Here's how the part is built. I have some questions about the finished solid (model axes, mm). A direction names the side the tool comes from. Round coordinates to 2 decimals unless told otherwise and drop trailing zeros. Loops run counter-clockwise (first coordinate to the right, second up) from the corner with the lowest first, then second, coordinate; pieces in that order, holes last. Notation, with made-up numbers: M -18.75,10 L 28.25,10 A20 ccw 28.25,49 Z; hole C 19,1 d7. An arc over 180 degrees is marked long. Answer as a JSON object with one key per item and string values.
Autodesk Inventor part; units mm, degrees
ref_plane "YZ Plane" through (0, 0, 0) normal (1, 0, 0) x (0, 1, 0)
ref_plane "XZ Plane" through (0, 0, 0) normal (0, 1, 0) x (-1, 0, 0)
ref_plane "XY Plane" through (0, 0, 0) normal (0, 0, 1) x (1, 0, 0)
sketch "Sketch1" plane through (0, 0, 0) normal (0, 0, 1) x (1, 0, 0)
  line L0 (0, 0) -> (55, 0)
  line L1 (55, 0) -> (55, 10)
  line L2 (55, 10) -> (0, 10)
  line L3 (0, 10) -> (0, 0)
  dimension "d0" = 55
  dimension "d1" = 10
extrude "Extrusion1" add sketch "Sketch1" along normal blind 3.175
sketch "Sketch3" plane through (0, 0, 3.175) normal (0, 0, 1) x (1, 0, 0)
  line L0 (37, 5) -> (55, 5)
  line L1 (0, 10) -> (55, 10)
  line L2 (0, 0) -> (6, 0) construction
  line L3 (6, 0) -> (6, 10) construction
  line L4 (6, 10) -> (0, 10) construction
  line L5 (0, 10) -> (0, 0) construction
  line L6 (-4.3576, 5) -> (33.1549, 5) construction
  line L7 (6, 0) -> (28.9, 0) construction
  line L8 (28.9, 0) -> (28.9, 6.8677) construction
  line L9 (28.9, 6.8677) -> (6, 6.8677) construction
  line L10 (6, 6.8677) -> (6, 0) construction
  point P0 (6, 5)
  point P1 (28.9, 5)
  dimension "d8" = 6
  dimension "d9" = 22.9
hole "Hole1" at (6, 5, 3.175) at (28.9, 5, 3.175) direction (0, 0, -1) diameter 3.2 end through all
sketch "Sketch6" plane through (0, 0, 3.175) normal (0, 0, 1) x (1, 0, 0)
  line L0 (55, 10) -> (37, 10)
  line L1 (37, 10) -> (37, 5)
  line L2 (37, 5) -> (55, 5)
  line L3 (55, 5) -> (55, 10)
  dimension "d32" = 18
  dimension "d33" = 5
extrude "Extrusion4" add sketch "Sketch6" along normal blind 10
sketch "Sketch7" plane through (37, 5, 3.175) normal (0, -1, 0) x (1, 0, 0)
  line L0 (18, 0) -> (18, 10)
  line L1 (9, 13.1417) -> (9, -6.2593) construction
  line L2 (-2.325, 5) -> (23.2178, 5) construction
  point P0 (-37, -3.175)
  point P1 (9, 5)
hole "Hole3" at (46, 5, 8.175) direction (0, 1, 0) diameter 3 end through all
thread "Thread2"
sketch "Sketch8" plane through (55, 0, 0) normal (1, 0, 0) x (0, 0, -1)
  line L0 (-3.175, 5) -> (-13.175, 5)
  line L1 (-13.175, 5) -> (-12.775, 5) construction
  line L2 (-12.775, 5) -> (-12.775, 5.2) construction
  line L3 (-12.775, 5.2) -> (-13.175, 5.2) construction
  line L4 (-13.175, 5.2) -> (-13.175, 5) construction
  line L5 (-12.775, 5.2) -> (-12.575, 5)
  line L6 (-12.775, 5.2) -> (-12.4922, 5.2) construction
  line L7 (-12.775, 5.2) -> (-12.975, 5)
  line L8 (-12.775, 5.2) -> (-12.4922, 5.2) construction
  line L9 (-12.975, 5) -> (-12.575, 5)
  dimension "d45" = 0.4
  dimension "d46" = 0.2
  dimension "d47" = 45
  dimension "d48" = 135
extrude "Extrusion5" cut sketch "Sketch8" against normal through all
properties part number "alpha_omega_holder"
Item 1: I want a section at D-D on x = 46. List the corners of the cut face in (y, z) for me (3 decimals).
Solution:
{"outline": "M 0,0 L 10,0 L 10,6.675 L 5,6.675 L 5,3.175 L 0,3.175 Z; M 5,9.675 L 10,9.675 L 10,13.175 L 5,13.175 L 5,12.975 L 5.2,12.775 L 5,12.575 Z"}
Item 2: For P1, Ø2.5, axis at y = 7.5, z = 8.5, coming from the -X side; P2, Ø3, axis at x = 16.5, y = 6.5, coming from the +Z side (3 decimals); P3, Ø2.5, axis at x = 46, z = 8.175, coming from the +Y side; P4, Ø1, axis at x = 37, z = 9, coming from the -Y side, each with a flat end and sliding along its axis, tell me the tip position at first contact or that it passes through.
Solution:
{"P1": "stops at x = 37", "P2": "stops at z = 3.175", "P3": "passes through", "P4": "stops at y = 5"}
Item 3: I want a section at A-A on x = 6. List the corners of the cut face in (y, z) for me (3 decimals), plus the area to 3 significant figures.
Solution:
{"outline": "M 0,0 L 3.4,0 L 3.4,3.175 L 0,3.175 Z; M 6.6,0 L 10,0 L 10,3.175 L 6.6,3.175 Z", "area": "21.6 mm2"}
Item 4: For faces 4 (the face through (0, 5, 2)), 5 (the face through (44, 5, 8)), which set-ups out of +Z, -Z, +X, -X, +Y, -Y let a thin tool reach every point of the face, with its end or its side?
Solution:
{"face 4": "+Z, -Z, -X, +Y, -Y", "face 5": "+Z, +X, -X, -Y"}
Item 5: I want a section at C-C on z = 7.5. List the corners of the cut face in (x, y) for me, plus the area to 3 significant figures.
Solution:
{"outline": "M 37,5 L 44.66,5 L 44.66,10 L 37,10 Z; M 47.34,5 L 55,5 L 55,10 L 47.34,10 Z", "area": "76.6 mm2"}
Item 6: I want a section at B-B on y = 7.5. List the corners of the cut face in (x, z) for me (3 decimals), plus the area to 3 significant figures.
Solution:
{"outline": "M 0,0 L 55,0 L 55,13.175 L 37,13.175 L 37,3.175 L 0,3.175 Z; hole C 46,8.175 d3", "area": "348 mm2"}
Item 7: We'd pull the mould along X, two halves only. Please class faces 1 (the face through (37, 8, 8)), 2 (the face through (47.464, 7.535, 8.5)), 3 (the face through (40, 10, 5)): +X half, -X half, draft (parallel to the pull), parting line (faces both ways), or undercut.
Solution:
{"face 1": "-X half", "face 2": "undercut", "face 3": "draft"}
Item 8: If I drill on L1, parallel to X at y = 5, z = 0.75; L2, parallel to Z at x = 46, y = 6.35 (3 decimals); L3, parallel to Y at x = 6, z = 2.25, over which ranges is the centre line in solid material (lowest first)? Write a range as from..to.
Solution:
{"L1": "x = 0..4.4, 7.6..27.3, 30.5..55", "L2": "z = 0..6.675, 9.675..13.175", "L3": "y = 0..3.4, 6.6..10"}
